from build123d import *

# Parameters (mm, degrees)
SKETCH1_R               = 37.5
BOSS_EXTRUDE1_DEPTH     = 75
SKETCH2_R               = 31.5
BOSS_EXTRUDE2_DEPTH     = 6.5
SKETCH3_R               = 15.75
CUT_EXTRUDE1_DEPTH      = 6.5
SKETCH4_R               = 3
CUT_EXTRUDE2_DEPTH      = 5
BOSS_EXTRUDE3_START     = -10
BOSS_EXTRUDE3_DEPTH     = 6
CUT_EXTRUDE4_REACH      = 123.333
CUT_EXTRUDE4_END_RADIUS = 37.5
SKETCH7_R               = 7.955992876
SKETCH7_R_2             = 3


with BuildPart() as part:
    # Sketch1 → Boss-Extrude1 (new body)
    with BuildSketch(Plane.XY):
        Circle(SKETCH1_R)
    extrude(amount=BOSS_EXTRUDE1_DEPTH)

    # Sketch2 → Boss-Extrude2 (add)
    with BuildSketch(Plane(origin=(0, 0, 0), x_dir=(-1, 0, 0), z_dir=(0, 0, -1))):
        with Locations(Location((0, 0, 0), (0, 0, 180))):
            Circle(SKETCH2_R)
    extrude(amount=BOSS_EXTRUDE2_DEPTH)

    # Sketch3 → Cut-Extrude1 (cut)
    with BuildSketch(Plane(origin=(0, 0, -6.5), x_dir=(-1, 0, 0), z_dir=(0, 0, -1))):
        Circle(SKETCH3_R)
    extrude(amount=-CUT_EXTRUDE1_DEPTH, mode=Mode.SUBTRACT)

    # Sketch4 → Cut-Extrude2 (cut)
    with BuildSketch(Plane(origin=(0, 0, -6.5), x_dir=(-1, 0, 0), z_dir=(0, 0, -1))):
        with Locations((25, 0)):
            Circle(SKETCH4_R)
        with Locations((0, -25)):
            Circle(SKETCH4_R)
        with Locations((-25, 0)):
            Circle(SKETCH4_R)
        with Locations((0, 25)):
            Circle(SKETCH4_R)
    extrude(amount=-CUT_EXTRUDE2_DEPTH, mode=Mode.SUBTRACT)

    # Sketch6 → Boss-Extrude3 (add)
    with BuildSketch(Plane(origin=(0, 0, 0), x_dir=(-1, 0, 0), z_dir=(0, 0, -1)).offset(BOSS_EXTRUDE3_START)):
        with BuildLine():
            ThreePointArc((-24.310194937, -28.552835624), (-25.433737437, -27.556759606), (-26.516504294, -26.516504294))
            Line((-26.516504294, -26.516504294), (-29.941404236, -29.941404236))
            Line((-29.941404236, -29.941404236), (-27.820083892, -32.062724579))
            Line((-27.820083892, -32.062724579), (-24.310194936, -28.552835624))
        make_face()
        with BuildLine():
            Line((-29.941404236, -29.941404236), (-26.516504294, -26.516504294))
            ThreePointArc((-26.516504294, -26.516504294), (-27.556759606, -25.433737437), (-28.552835624, -24.310194937))
            Line((-28.552835624, -24.310194936), (-32.062724579, -27.820083892))
            Line((-32.062724579, -27.820083892), (-29.941404236, -29.941404236))
        make_face()
    extrude(amount=-BOSS_EXTRUDE3_DEPTH)

    # Cut-Extrude4: up to this cylinder (the profile starts outside it)
    cut_extrude4_end = Plane(origin=(0, 0, 20.730963), z_dir=(0, 0, -1)) * Cylinder(CUT_EXTRUDE4_END_RADIUS, 322.666, mode=Mode.PRIVATE)
    # Sketch7 → Cut-Extrude4 (cut, up to the surface)
    with BuildSketch(Plane(origin=(29.941404236, -29.941404236, 0), x_dir=(0, 0, -1), z_dir=(0.7071067811865471, -0.7071067811865479, 0)), mode=Mode.PRIVATE) as cut_extrude4_sk1:
        with Locations((-13, 0)):
            Circle(SKETCH7_R)
        with Locations(Location((-13, 0, 0), (0, 0, 90))):
            Circle(SKETCH7_R_2, mode=Mode.SUBTRACT)
    cut_extrude4_tool1 = extrude(cut_extrude4_sk1.sketch, amount=-CUT_EXTRUDE4_REACH, mode=Mode.PRIVATE) - cut_extrude4_end
    add(cut_extrude4_tool1.solids().sort_by_distance((29.941404, -29.941404, 20.730963))[0], mode=Mode.SUBTRACT)


solid = part.part
Here's how the part is built. I have some questions about the finished solid (model axes, mm). A direction names the side the tool comes from. Give positions to 0.01 mm unless a question says otherwise; leave off trailing zeros. Order: outer loops, then holes, each group sorted by start corner. A loop starts at its lowest first (then second) coordinate and runs counter-clockwise, first axis right, second up. Notation, with made-up numbers: M 19.25,69 L 44.25,69 A33 cw 44.25,100 Z; hole C 61.5,19.25 d6. An arc over 180 degrees is marked long. Answer as a JSON object with one key per item and string values. Group by question number.
1) Suppose I cut it at D-D, the plane x = 11. Write out the boundary of the cut face in (y, z).
2) On a 3-axis mill with a long thin cutter (end or side, diameter ignored), from which of +Z, -Z, +X, -X, +Y, -Y can I reach the whole of each face in a straight line? I mean faces 1 (the cylindrical face through (28, 0, -4)), 2 (the cylindrical face through (30, -26, 12)). Say none if no direction works.
3) Suppose I cut it at C-C, the plane z = 23. Write out the boundary of the cut face in (x, y).
4) We'd pull the mould along Y, two halves only. Please class faces 3 (the cylindrical face through (-4.101, -31.232, -3.204)), 4 (the flat face through (-1, 1, 75)), 5 (the flat face through (-25, 0, -1.5)): pulls with the +Y half, pulls with the -Y half, needs draft (parallel to the pull), parting line crosses it, or undercut.
5) Please list where these lines run through material, in increasing order: L1, parallel to Y at x = 0, z = -4; L2, parallel to Z at x = -10, y = -6; L3, parallel to X at y = 0.5, z = 43. Write a range as [from, to].
6) Suppose I cut it at A-A, the plane y = 0. Write out the boundary of the cut face in (x, z), plus the area to 3 significant figures.
7) I'm going to push flat-ended pins straight in: pin 1 Ø16 at (x, y) = (7.5, 1.5) entering from -Z; pin 2 Ø3.5 at (x, y) = (0, -25) entering from -Z; pin 3 Ø1.5 at (x, z) = (1.5, 14.5) entering from -Y. Where does each tip first touch, or does it pass through?
Results found:
{
 "1": {"outline": "M -35.85,0 L -29.52,0 L -29.52,-6.5 L -11.27,-6.5 L -11.27,0 L 11.27,0 L 11.27,-6.5 L 29.52,-6.5 L 29.52,0 L 35.85,0 L 35.85,75 L -35.85,75 Z"},
 "2": {"face 1": "-Z", "face 2": "none"},
 "3": {"outline": "C 0,0 d75"},
 "4": {"face 3": "parting line crosses it", "face 4": "needs draft", "face 5": "undercut"},
 "5": {"L1": "[-31.5, -28], [-22, -15.75], [15.75, 22], [28, 31.5]", "L2": "[0, 75]", "L3": "[-37.5, 37.5]"},
 "6": {"outline": "M -37.5,0 L -31.5,0 L -31.5,-6.5 L -28,-6.5 L -28,-1.5 L -22,-1.5 L -22,-6.5 L -15.75,-6.5 L -15.75,0 L 15.75,0 L 15.75,-6.5 L 22,-6.5 L 22,-1.5 L 28,-1.5 L 28,-6.5 L 31.5,-6.5 L 31.5,0 L 37.5,0 L 37.5,75 L -37.5,75 Z", "area": "5,770 mm²"},
 "7": {"pin 1": "z = 0", "pin 2": "z = -1.5", "pin 3": "y = -37.49"}
}
